The model under review builds one solid part; all positions refer to its coordinate system, in mm. A direction names the side the tool comes from. Round coordinates to 2 decimals unless told otherwise and drop trailing zeros. Loops run counter-clockwise (first coordinate to the right, second up) from the corner with the lowest first, then second, coordinate; pieces in that order, holes last. Notation, with made-up numbers: (28, 0.5) -> (53, 0.5) arc R5 cw to (53, 6.5) -> close; hole circle Ø9 at (33, 17.5). An arc over 180 degrees is marked (long way). Write each question's results on one line, items separated by ' | '. Start each with the question number.
Item 1: Mouldability with a two-part tool opening along Y and no side actions: class faces 1 (the cylindrical face through (13.498, 40.395, 36.22)), 2 (the flat face through (19, -28, 0)) as pulls with the +Y half, pulls with the -Y half, needs draft (parallel to the pull), parting line crosses it, or undercut.
Item 2: For L1, parallel to Z at x = 32.3, y = -32; L2, parallel to X at y = 46, z = 55.5; L3, parallel to X at y = -1, z = 32, list the stretches that pass through material, from the lowest coordinate up. Write a range as from..to.
Item 3: We need section C-C (y = 35.5). Give the boundary of the cut face in (x, z), and give its area (3 significant figures).
Item 4: We need section A-A (y = -31). Give the boundary of the cut face in (x, z).
Item 5: Tool access review of faces 3 (the cylindrical face through (17.6, -35.89, 36)), 4 (the flat face through (38, -39, 58.9)), 5 (the cylindrical face through (-10.33, -40.93, 38.53)): name each direction out of +Z, -Z, +X, -X, +Y, -Y from which nothing blocks a thin tool from reaching the whole face with its end or side.
Item 6: Clearance check with flat-ended pins moving along their axes: pin 1 Ø8 at (x, z) = (-32.3, 9) entering from +Y; pin 2 Ø9 at (x, z) = (-40.5, 37) entering from +Y; pin 3 Ø8 at (y, z) = (45.39, 36) entering from +X. State where each tip first meets the part, or that it passes through.
Item 7: We need section B-B (x = -37). Give the boundary of the cut face in (y, z).
from build123d import *

# Parameters (mm, degrees)
F1_DEPTH       = 72
F2_R           = 2.55
F3_DEPTH       = 25
F4_R           = 2.55
F5_DEPTH       = 10
F6_R           = 3
F7_R           = 3
F8_R           = 3
F9_R           = 2
F10_DEPTH      = 25
F10_DEPTH_BACK = 25
F13_R          = 5
F14_DEPTH      = 15
F15_R          = 5
F16_DEPTH      = 15
F18_DEPTH      = 5.5
F19_R          = 3
F20_R          = 1


with BuildPart() as f1:
    # F0 (on Top) → F1 (new body)
    with BuildSketch(Plane.XY):
        with BuildLine():
            Line((-41.897575, -9.674357), (-45, -16))
            Line((-45, -16), (-45, -45))
            Line((-45, -45), (45, -45))
            Line((45, -45), (45, -16))
            Line((45, -16), (41.897575, -9.674357))
            ThreePointArc((41.897575, -9.674357), (39.104117, 17.884855), (20.082904, 38.022059))
            Line((20.082904, 38.022059), (12, 52.022059))
            Line((12, 52.022059), (2, 52.022059))
            Line((2, 52.022059), (2, 32.939338))
            ThreePointArc((2, 32.939338), (31.828637, 8.714233), (18.5, -27.326727))
            Line((18.5, -27.326727), (18.5, -36.75))
            Line((18.5, -36.75), (-18.5, -36.75))
            Line((-18.5, -36.75), (-18.5, -27.326727))
            ThreePointArc((-18.5, -27.326727), (-31.828637, 8.714233), (-2, 32.939338))
            Line((-2, 32.939338), (-2, 52.022059))
            Line((-2, 52.022059), (-12, 52.022059))
            Line((-12, 52.022059), (-20.082904, 38.022059))
            ThreePointArc((-20.082904, 38.022059), (-39.104117, 17.884855), (-41.897575, -9.674357))
        make_face()
    extrude(amount=F1_DEPTH)

    # F2 (on face) → F3 (cut)
    with BuildSketch(Plane.XZ.offset(45)):
        with Locations((-32.3, 9)):
            Circle(F2_R)
        with Locations((-10, 9)):
            Circle(F2_R)
        with Locations((10, 9)):
            Circle(F2_R)
        with Locations((32.3, 9)):
            Circle(F2_R)
        with Locations((32.3, 36)):
            Circle(F2_R)
        with Locations((10, 36)):
            Circle(F2_R)
        with Locations((-10, 36)):
            Circle(F2_R)
        with Locations((-32.3, 36)):
            Circle(F2_R)
        with Locations((-32.3, 63)):
            Circle(F2_R)
        with Locations((-10, 63)):
            Circle(F2_R)
        with Locations((10, 63)):
            Circle(F2_R)
        with Locations((32.3, 63)):
            Circle(F2_R)
    extrude(amount=-F3_DEPTH, mode=Mode.SUBTRACT)

    # F4 (on face) → F5 (cut)
    with BuildSketch(Plane(origin=(0, 0, 0), x_dir=(1, 0, 0), z_dir=(0, 0, -1))):
        with Locations((-37, 16)):
            Circle(F4_R)
        with Locations((37, 16)):
            Circle(F4_R)
    extrude(amount=-F5_DEPTH, mode=Mode.SUBTRACT)

    # F6
    f6_edges = [f1.edges().sort_by_distance(p)[0] for p in [
        (18.5, -27.326727, 36),
        (18.5, -36.75, 36),
        (-18.5, -27.326727, 36),
        (-18.5, -36.75, 36),
    ]]
    fillet(f6_edges, radius=F6_R)

    # F7
    f7_edges = [f1.edges().sort_by_distance(p)[0] for p in [
        (-41.897575, -9.674357, 36),
        (-45, -16, 36),
        (41.897575, -9.674357, 36),
        (45, -16, 36),
    ]]
    fillet(f7_edges, radius=F7_R)

    # F8
    f8_edges = [f1.edges().sort_by_distance(p)[0] for p in [
        (-20.082904, 38.022059, 36),
        (20.082904, 38.022059, 36),
    ]]
    fillet(f8_edges, radius=F8_R)

    # F9 (on Right) → F10 (cut, two sides)
    with BuildSketch(Plane.YZ) as f10_sk:
        with Locations((45.389666, 58.5)):
            Circle(F9_R)
        with Locations((45.389666, 36)):
            Circle(F9_R)
        with Locations((45.389666, 13.5)):
            Circle(F9_R)
    extrude(amount=F10_DEPTH, mode=Mode.SUBTRACT)
    extrude(f10_sk.sketch, amount=-F10_DEPTH_BACK, mode=Mode.SUBTRACT)

    # F13 (on offset) → F14 (cut)
    with BuildSketch(Plane.YZ.offset(25)):
        with Locations((45.389666, 58.5)):
            Circle(F13_R)
        with Locations((45.389666, 36)):
            Circle(F13_R)
        with Locations((45.389666, 13.5)):
            Circle(F13_R)
    extrude(amount=-F14_DEPTH, mode=Mode.SUBTRACT)

    # F15 (on offset) → F16 (cut)
    with BuildSketch(Plane.YZ.offset(-25)):
        with Locations((45.389666, 58.5)):
            Circle(F15_R)
        with Locations((45.389666, 36)):
            Circle(F15_R)
        with Locations((45.389666, 13.5)):
            Circle(F15_R)
    extrude(amount=F16_DEPTH, mode=Mode.SUBTRACT)

    # F17 (on face) → F18 (cut)
    with BuildSketch(Plane(origin=(0, -36.75, 0), x_dir=(-1, 0, 0), z_dir=(0, 1, 0))):
        Polygon((27.565728, 36), (29.932864, 31.9), (34.667136, 31.9), (54.795958, 31.9), (54.795958, 40.1), (34.667136, 40.1), (29.932864, 40.1), align=None)
        Polygon((27.565728, 63), (29.932864, 58.9), (34.667136, 58.9), (54.795958, 58.9), (54.795958, 67.1), (34.667136, 67.1), (29.932864, 67.1), align=None)
        Polygon((27.565728, 9), (29.932864, 4.9), (34.667136, 4.9), (54.795958, 4.9), (54.795958, 13.1), (34.667136, 13.1), (29.932864, 13.1), align=None)
        Polygon((-29.932864, 13.1), (-34.667136, 13.1), (-55.134665, 13.1), (-55.134665, 4.9), (-34.667136, 4.9), (-29.932864, 4.9), (-27.565728, 9), align=None)
        Polygon((-29.932864, 40.1), (-34.667136, 40.1), (-55.134665, 40.1), (-55.134665, 31.9), (-34.667136, 31.9), (-29.932864, 31.9), (-27.565728, 36), align=None)
        Polygon((-29.932864, 67.1), (-34.667136, 67.1), (-55.134665, 67.1), (-55.134665, 58.9), (-34.667136, 58.9), (-29.932864, 58.9), (-27.565728, 63), align=None)
    extrude(amount=-F18_DEPTH, mode=Mode.SUBTRACT)

    # F19
    f19_edges = [f1.edges().sort_by_distance(p)[0] for p in [
        (-12, 52.022059, 36),
        (12, 52.022059, 36),
    ]]
    fillet(f19_edges, radius=F19_R)

    # F20
    f20_edges = [f1.edges().sort_by_distance(p)[0] for p in [
        (2, 32.939338, 36),
        (-2, 32.939338, 36),
        (31.624924, 9.426781, 72),
    ]]
    fillet(f20_edges, radius=F20_R)


solid = f1.part
Here are the results:
1) face 1: undercut | face 2: needs draft
2) L1: z = 0..6.45, 11.55..33.45, 38.55..60.45, 65.55..72 | L2: x = -10..-2, 2..10 | L3: x = -42.99..-32.98, 32.98..42.99
3) outline: (-24.26, 0) -> (-2, 0) -> (-2, 72) -> (-24.26, 72) -> close; (2, 0) -> (24.26, 0) -> (24.26, 72) -> (2, 72) -> close | area: 3,210 mm2
4) outline: (-45, 0) -> (-18.5, 0) -> (-18.5, 71) arc R1 ccw to (-19.5, 72) -> (-45, 72) -> close; (18.5, 0) -> (45, 0) -> (45, 72) -> (19.5, 72) arc R1 ccw to (18.5, 71) -> close; hole circle Ø5.1 at (-32.3, 9); hole circle Ø5.1 at (-32.3, 36); hole circle Ø5.1 at (-32.3, 63); hole circle Ø5.1 at (32.3, 9); hole circle Ø5.1 at (32.3, 36); hole circle Ø5.1 at (32.3, 63)
5) face 3: +Z, -Z | face 4: +X | face 5: -Y
6) pin 1: stops at y = 32.37 | pin 2: stops at y = 23.52 | pin 3: stops at x = 10
7) outline: (-45, 0) -> (-18.55, 0) -> (-18.55, 10) -> (-13.45, 10) -> (-13.45, 0) -> (21.91, 0) -> (21.91, 72) -> (-45, 72) -> close; hole (-42.25, 4.9) -> (-36.75, 4.9) -> (-36.75, 13.1) -> (-42.25, 13.1) -> close; hole (-42.25, 31.9) -> (-36.75, 31.9) -> (-36.75, 40.1) -> (-42.25, 40.1) -> close; hole (-42.25, 58.9) -> (-36.75, 58.9) -> (-36.75, 67.1) -> (-42.25, 67.1) -> close
